from build123d import *

# Parameters (mm, degrees)
CYLINDER005_R     = 51
CYLINDER005_DEPTH = 20
CYLINDER004_R     = 70.0875
CYLINDER004_DEPTH = 20


with BuildPart() as cylinder005:
    # Cylinder005 → Cylinder005 (new body)
    with BuildSketch(Plane(origin=(105, 68, 0), x_dir=(1, 0, 0), z_dir=(0, 0, 1))):
        Circle(CYLINDER005_R)
    extrude(amount=CYLINDER005_DEPTH)


with BuildPart() as inlet:
    # Cylinder004 → Cylinder004 (new body)
    with BuildSketch(Plane(origin=(105, 148, 0), x_dir=(1, 0, 0), z_dir=(0, 0, 1))):
        Circle(CYLINDER004_R)
    extrude(amount=CYLINDER004_DEPTH)

    # Common: intersect Cylinder005
    add(cylinder005.part, mode=Mode.INTERSECT)


solid = inlet.part
Check sheet for the modelled part. Datum: model origin and axes. Units: mm. Coordinates: 2 decimals unless noted, no trailing zeros. Write each loop counter-clockwise with the first axis right and the second up, starting at its lowest first coordinate (ties: lowest second). Pieces come first, ordered by that corner, then holes. Notation, with made-up numbers: M -32.5,-17 L -3.5,-17 A22 ccw -3.5,21 Z; hole C 84.25,45 d7. An arc over 180 degrees is marked long. Answer as CSV lines item,"result".
Q1. Cross-section at C-C (y = 102.5). Record the boundary of the cut face in (x, z), then the cut area to 3 significant figures.
Check result:
outline,"M 67.44,0 L 142.56,0 L 142.56,20 L 67.44,20 Z"
area,"1,500 mm^2"
Q2. Go/stop test with flat-tipped pins: pin 1 (1.5 mm diameter, centred on y = 103, z = 8, fed in from +X); pin 2 (4 mm diameter, centred on y = 83, z = 2.5, fed in from +X); pin 3 (8 mm diameter, centred on x = 98.5, z = 14, fed in from +Y). Record where each tip stops, or that it passes through.
Check result:
pin 1,"x = 142.79"
pin 2,"x = 135.71"
pin 3,"y = 118.94"
Q3. Cross-section at B-B (x = 87). Record the boundary of the cut face in (y, z), then the cut area to 3 significant figures.
Check result:
outline,"M 80.26,0 L 115.72,0 L 115.72,20 L 80.26,20 Z"
area,"709 mm^2"
Q4. Cross-section at A-A (z = 10.5). Record the boundary of the cut face in (x, y) (1 decimal).
Check result:
outline,"M 60.9,93.6 A70.1 ccw 149.1,93.6 A51 ccw Z"
Q5. Material ranges on probe 1 along Y at (x, z) = (104.5, 16.5); probe 2 along Y at (x, z) = (97, 7); probe 3 along X at (y, z) = (88, 15), recorded low to high. Write a range as from..to.
Check result:
probe 1,"77.91..119"
probe 2,"78.37..118.37"
probe 3,"68.77..141.23"
